from build123d import *

# Parameters (mm, degrees)
SKETCH1_W           = 5
SKETCH1_H           = 5
SKETCH1_R           = 1.5
SKETCH1_R_2         = 1.25
BOSS_EXTRUDE1_DEPTH = 5


with BuildPart() as part:
    # Sketch1 → Boss-Extrude1 (new body)
    with BuildSketch(Plane.XY):
        Polygon((-50, 65), (-50, -65), (-35, -65), (-35, -68), (-30, -68), (-30, -65), (-26.5, -65), (-26.5, -62), (-27.6, -62), (-27.6, -59.7), (-26.5, -59.7), (-26.5, -55), (-23.5, -55), (-23.5, -59.7), (-22.4, -59.7), (-22.4, -62), (-23.5, -62), (-23.5, -65), (-20, -65), (-20, -68), (-15, -68), (-15, -65), (15, -65), (15, -68), (20, -68), (20, -65), (23.5, -65), (23.5, -62), (22.4, -62), (22.4, -59.7), (23.5, -59.7), (23.5, -55), (26.5, -55), (26.5, -59.7), (27.6, -59.7), (27.6, -62), (26.5, -62), (26.5, -65), (30, -65), (30, -68), (35, -68), (35, -65), (50, -65), (50, 65), (35, 65), (35, 70), (30, 70), (30, 65), (26.5, 65), (26.5, 62), (27.6, 62), (27.6, 59.7), (26.5, 59.7), (26.5, 55), (23.5, 55), (23.5, 59.7), (22.4, 59.7), (22.4, 62), (23.5, 62), (23.5, 65), (20, 65), (20, 70), (15, 70), (15, 65), (-15, 65), (-15, 70), (-20, 70), (-20, 65), (-23.5, 65), (-23.5, 62), (-22.4, 62), (-22.4, 59.7), (-23.5, 59.7), (-23.5, 55), (-26.5, 55), (-26.5, 59.7), (-27.6, 59.7), (-27.6, 62), (-26.5, 62), (-26.5, 65), (-30, 65), (-30, 70), (-35, 70), (-35, 65), align=None)
        with Locations((-42.5, -54)):
            Rectangle(SKETCH1_W, SKETCH1_H, mode=Mode.SUBTRACT)
        with Locations((-42.5, -46.5)):
            Circle(SKETCH1_R, mode=Mode.SUBTRACT)
        with Locations((-42.5, -39)):
            Rectangle(SKETCH1_W, SKETCH1_H, mode=Mode.SUBTRACT)
        with Locations((-42.5, -7.5)):
            Rectangle(SKETCH1_W, SKETCH1_H, mode=Mode.SUBTRACT)
        with Locations((-42.5, 0)):
            Circle(SKETCH1_R, mode=Mode.SUBTRACT)
        with Locations((42.5, -54)):
            Rectangle(SKETCH1_W, SKETCH1_H, mode=Mode.SUBTRACT)
        with Locations((42.5, -46.5)):
            Circle(SKETCH1_R, mode=Mode.SUBTRACT)
        with Locations((42.5, -39)):
            Rectangle(SKETCH1_W, SKETCH1_H, mode=Mode.SUBTRACT)
        with Locations((42.5, -7.5)):
            Rectangle(SKETCH1_W, SKETCH1_H, mode=Mode.SUBTRACT)
        with Locations((42.5, 0)):
            Circle(SKETCH1_R, mode=Mode.SUBTRACT)
        with Locations((-42.5, 7.5)):
            Rectangle(SKETCH1_W, SKETCH1_H, mode=Mode.SUBTRACT)
        with Locations((-31.819805153, 28.176796564)):
            Circle(SKETCH1_R_2, mode=Mode.SUBTRACT)
        with Locations((-42.5, 39)):
            Rectangle(SKETCH1_W, SKETCH1_H, mode=Mode.SUBTRACT)
        with Locations((-42.5, 46.5)):
            Circle(SKETCH1_R, mode=Mode.SUBTRACT)
        with Locations((-42.5, 54)):
            Rectangle(SKETCH1_W, SKETCH1_H, mode=Mode.SUBTRACT)
        with Locations((-21.213203436, 38.783398282)):
            Circle(SKETCH1_R_2, mode=Mode.SUBTRACT)
        with Locations((-10.606601718, 49.39)):
            Circle(SKETCH1_R_2, mode=Mode.SUBTRACT)
        with Locations((42.5, 7.5)):
            Rectangle(SKETCH1_W, SKETCH1_H, mode=Mode.SUBTRACT)
        with Locations((31.819805153, 28.176796564)):
            Circle(SKETCH1_R_2, mode=Mode.SUBTRACT)
        with Locations((10.606601718, 49.39)):
            Circle(SKETCH1_R_2, mode=Mode.SUBTRACT)
        with Locations((21.213203436, 38.783398282)):
            Circle(SKETCH1_R_2, mode=Mode.SUBTRACT)
        with Locations((42.5, 39)):
            Rectangle(SKETCH1_W, SKETCH1_H, mode=Mode.SUBTRACT)
        with Locations((42.5, 46.5)):
            Circle(SKETCH1_R, mode=Mode.SUBTRACT)
        with Locations((42.5, 54)):
            Rectangle(SKETCH1_W, SKETCH1_H, mode=Mode.SUBTRACT)
    extrude(amount=BOSS_EXTRUDE1_DEPTH)


solid = part.part
CAD build for the part. Positions are in the model's coordinates, mm. A direction names the side the tool comes from. Coordinates: 2 decimals unless noted, no trailing zeros. Order: outer loops, then holes, each group sorted by start corner. A loop starts at its lowest first (then second) coordinate and runs counter-clockwise, first axis right, second up. Notation, with made-up numbers: (-27, -6) -> (-23, -6) arc R27 ccw to (-23, 20) -> close; hole circle Ø2 at (8, -4.75). An arc over 180 degrees is marked (long way). Answer in a Markdown table with one row per item.
1) Which spindle directions (+Z, -Z, +X, -X, +Y, -Y) get a long thin tool onto all of the face, cutting with end or side? Do faces 4 (the face through (40, -54, 2)), 5 (the face through (-26.5, 63, 2)), 6 (the face through (-42, 65, 2)), 7 (the face through (23.5, -57, 2)). Say none if no direction does.
Check values:
| item | result |
|---|---|
| face 4 | +Z, -Z |
| face 5 | +Z, -Z, +Y |
| face 6 | +Z, -Z, -X, +Y |
| face 7 | +Z, -Z, -Y |
2) Flat gauge pins, fed straight in: P1, Ø1.2, axis at x = 23, z = 3.5, coming from the -Y side; P2, Ø1.5, axis at x = -41.5, z = 2.5, coming from the +Y side; P3, Ø1.5, axis at y = -66, z = 2, coming from the -X side. Where does each tip first touch, or does it go through?
Check values:
| item | result |
|---|---|
| P1 | y = -65 |
| P2 | y = 65 |
| P3 | x = -35 |
3) Band-saw the part on A-A (y = 0). List the corners of the cut face in (x, z).
Check values:
| item | result |
|---|---|
| outline | (-50, 0) -> (-44, 0) -> (-44, 5) -> (-50, 5) -> close; (-41, 0) -> (41, 0) -> (41, 5) -> (-41, 5) -> close; (44, 0) -> (50, 0) -> (50, 5) -> (44, 5) -> close |
4) Band-saw the part on B-B (x = 42.5). Give the number of separate pieces and of enclosed holes in the cut face, and give its area (3 significant figures).
Check values:
| item | result |
|---|---|
| separate pieces | 10 |
| enclosed holes | 0 |
| area | 455 mm2 |
5) Drill centre lines: line 1 (X direction, y = 58, z = 0.7); line 2 (Y direction, x = -27, z = 2.7); line 3 (X direction, y = 39, z = 2.2). Where is each one in solid material? Low to high.
Check values:
| item | result |
|---|---|
| line 1 | -50 to -26.5, -23.5 to 23.5, 26.5 to 50 |
| line 2 | -65 to -62, -59.7 to 59.7, 62 to 65 |
| line 3 | -50 to -45, -40 to -22.44, -19.98 to 19.98, 22.44 to 40, 45 to 50 |
6) Mould opens along Y. For faces 1 (the face through (15, 68, 2)), 2 (the face through (25, 55, 2)), 3 (the face through (45, -54, 2)) say: pulls with the +Y half, pulls with the -Y half, needs draft (parallel to the pull), parting line crosses it, or undercut.
Check values:
| item | result |
|---|---|
| face 1 | needs draft |
| face 2 | pulls with the +Y half |
| face 3 | undercut |
